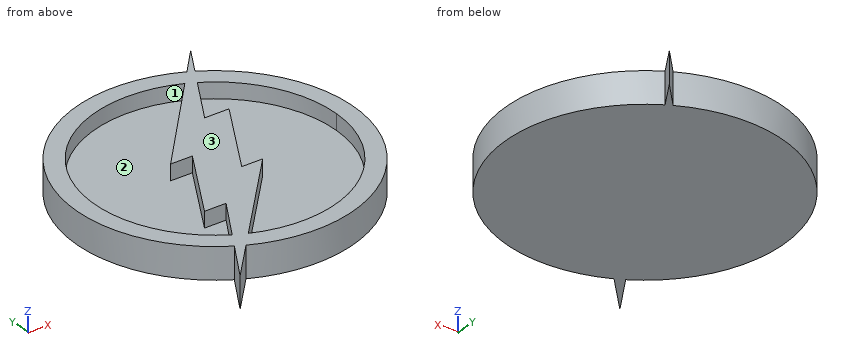
```python
from build123d import *

# Parameters (mm, degrees)
F1_DEPTH = 10.16
F2_DEPTH = 5.08


with BuildPart() as f1:
    # F0 (on Top) → F1 (new body)
    with BuildSketch(Plane.XY):
        with BuildLine():
            ThreePointArc((19.8948644209, 39.9997688602), (20.8320918018, 39.5197556971), (21.7577454104, 39.0177863782))
            Line((21.7577454104, 39.0177863782), (26.9711147994, 48.1350496411))
            Line((26.9711147994, 48.1350496411), (19.8948644209, 39.9997688602))
        make_face()
        with BuildLine():
            Line((-29.5520797372, -52.0064979792), (-19.2228405766, -40.327032365))
            ThreePointArc((-19.2228405766, -40.327032365), (-20.5915769431, -39.6456062912), (-21.9361932063, -38.9177410292))
            Line((-21.9361932063, -38.9177410292), (-29.5520797372, -52.0064979792))
        make_face()
        with BuildLine():
            ThreePointArc((-19.2228405766, -40.327032365), (23.8434631573, -37.7793118501), (44.6742335043, 0))
            ThreePointArc((44.6742335043, 0), (38.5214079324, 22.624947958), (21.7577454104, 39.0177863782))
            Line((21.7577454104, 39.0177863782), (18.8999443356, 34.0199965021))
            ThreePointArc((18.8999443356, 34.0199965021), (33.5418077285, 19.7361392424), (38.9174518423, 0))
            ThreePointArc((38.9174518423, 0), (21.4688277759, -32.460090755), (-15.2308770921, -35.8132439315))
            Line((-15.2308770922, -35.8132439315), (-19.2228405766, -40.327032365))
        make_face()
        with BuildLine():
            Line((18.8999443356, 34.0199965021), (21.7577454104, 39.0177863782))
            ThreePointArc((21.7577454104, 39.0177863782), (20.8320918018, 39.5197556971), (19.8948644209, 39.9997688602))
            Line((19.8948644209, 39.9997688602), (15.971442641, 35.4891684583))
            ThreePointArc((15.971442641, 35.4891684583), (17.4511611069, 34.7854140972), (18.8999443356, 34.0199965021))
        make_face()
        with BuildLine():
            ThreePointArc((-21.9361932063, -38.9177410292), (-20.5915769431, -39.6456062912), (-19.2228405766, -40.327032365))
            Line((-19.2228405766, -40.327032365), (-15.2308770922, -35.8132439315))
            ThreePointArc((-15.2308770921, -35.8132439315), (-17.1613070553, -34.9293228971), (-19.0406590573, -33.9414401662))
            Line((-19.0406590573, -33.9414401662), (-21.9361932063, -38.9177410292))
        make_face()
        with BuildLine():
            Line((9.9367275834, 18.344911789), (18.8999443356, 34.0199965021))
            ThreePointArc((18.8999443356, 34.0199965021), (17.4511611069, 34.7854140972), (15.971442641, 35.4891684583))
            Line((15.971442641, 35.4891684583), (-10.9691135585, 4.5166932978))
            Line((-10.9691135585, 4.5166932978), (-4.0004979819, 4.5166932978))
            Line((-4.0004979819, 4.5166932978), (-17.8778032411, -20.0695820685))
            Line((-17.8778032411, -20.0695820685), (-10.9691135585, -20.0695820685))
            Line((-10.9691135585, -20.0695820685), (-19.0406590573, -33.9414401662))
            ThreePointArc((-19.0406590573, -33.9414401662), (-17.1613070553, -34.9293228971), (-15.2308770921, -35.8132439315))
            Line((-15.2308770922, -35.8132439315), (9.9367275834, -7.3557584547))
            Line((9.9367275834, -7.3557584547), (3.2262078021, -7.3557584547))
            Line((3.2262078021, -7.3557584547), (17.7325143094, 18.344911789))
            Line((17.7325143094, 18.344911789), (9.9367275834, 18.344911789))
        make_face()
        with BuildLine():
            Line((15.971442641, 35.4891684583), (19.8948644209, 39.9997688602))
            ThreePointArc((19.8948644209, 39.9997688602), (-39.4719533034, 20.9225247427), (-21.9361932063, -38.9177410292))
            Line((-21.9361932063, -38.9177410292), (-19.0406590573, -33.9414401662))
            ThreePointArc((-19.0406590573, -33.9414401662), (-34.7492068376, 17.5231470361), (15.971442641, 35.4891684583))
        make_face()
    extrude(amount=F1_DEPTH)

    # F0 (on Top) → F2 (join)
    with BuildSketch(Plane.XY):
        with BuildLine():
            Line((-10.9691135585, 4.5166932978), (15.971442641, 35.4891684583))
            ThreePointArc((15.971442641, 35.4891684583), (-34.7492068376, 17.5231470361), (-19.0406590573, -33.9414401662))
            Line((-19.0406590573, -33.9414401662), (-10.9691135585, -20.0695820685))
            Line((-10.9691135585, -20.0695820685), (-17.8778032411, -20.0695820685))
            Line((-17.8778032411, -20.0695820685), (-4.0004979819, 4.5166932978))
            Line((-4.0004979819, 4.5166932978), (-10.9691135585, 4.5166932978))
        make_face()
        with BuildLine():
            ThreePointArc((38.9174518423, 0), (33.5418077285, 19.7361392424), (18.8999443356, 34.0199965021))
            Line((18.8999443356, 34.0199965021), (9.9367275834, 18.344911789))
            Line((9.9367275834, 18.344911789), (17.7325143094, 18.344911789))
            Line((17.7325143094, 18.344911789), (3.2262078021, -7.3557584547))
            Line((3.2262078021, -7.3557584547), (9.9367275834, -7.3557584547))
            Line((9.9367275834, -7.3557584547), (-15.2308770922, -35.8132439315))
            ThreePointArc((-15.2308770921, -35.8132439315), (21.4688277759, -32.460090755), (38.9174518423, 0))
        make_face()
    extrude(amount=F2_DEPTH)


solid = f1.part
```
Geometry check sheet. Reference: the model listing, model coordinates, mm. Face numbers are marked on the shaded views. Round coordinates to 2 decimals unless told otherwise and drop trailing zeros. Order: outer loops, then holes, each group sorted by start corner. A loop starts at its lowest first (then second) coordinate and runs counter-clockwise, first axis right, second up. Notation, with made-up numbers: (38.25, -31.5) - (81.25, -31.5) arc R24 cw to (81.25, -12.5) - close; hole circle Ø5 at (-16.75, 18). An arc over 180 degrees is marked (long way). Use a Markdown table: item, result. Add a question column.
(1) Release check for a two-part mould opening along X. For the marked faces 1, 2 and 3 record: pulls with the +X half, pulls with the -X half, needs draft (parallel to the pull), parting line crosses it, or undercut.
(2) Material ranges on line 1 along X through (y, z) = (-21.5, 7.25); line 2 along X through (y, z) = (6, 6.5); line 3 along Y through (x, z) = (14, 7.25), recorded low to high. Write a range as [from, to].
(3) Sectioned sample at D-D, the plane y = 29.5. Enter the section's corners in (x, z), and give its area (3 significant figures).
(4) Sectioned sample at B-B, the plane x = -24. Enter the section's corners in (y, z).
(5) Sectioned sample at C-C, the plane y = -43.5. Enter the section's corners in (x, z).
(6) Depth check by flat-ended pin: pin 1 (2.5 mm diameter, centred on x = 7, z = 7.5, fed in from +Y); pin 2 (1.5 mm diameter, centred on y = 12, z = 5.5, fed in from +X); pin 3 (1.5 mm diameter, centred on x = -8, z = 8, fed in from -Y); pin 4 (1 mm diameter, centred on x = 17.5, y = 21, fed in from -Z). Enter the tip coordinate at first touch or a pass-through.
Answers below:
| question | item | result |
|---|---|---|
| 1 | face 1 | undercut |
| 1 | face 2 | undercut |
| 1 | face 3 | needs draft |
| 2 | line 1 | [-39.16, -32.44], [-11.8, -2.57], [32.44, 39.16] |
| 2 | line 2 | [-44.27, -38.45], [-9.68, 10.76], [38.45, 44.27] |
| 2 | line 3 | [-42.42, -36.31], [11.73, 18.34], [25.45, 33.22], [36.31, 42.42] |
| 3 | outline | (-33.55, 0) - (33.55, 0) - (33.55, 10.16) - (25.38, 10.16) - (25.38, 5.08) - (16.32, 5.08) - (16.32, 10.16) - (10.76, 10.16) - (10.76, 5.08) - (-25.38, 5.08) - (-25.38, 10.16) - (-33.55, 10.16) - close |
| 3 | area | 452 mm² |
| 4 | outline | (-45.73, 0) - (-42.46, 0) - (-42.46, 10.16) - (-45.73, 10.16) - close; (-37.68, 0) - (37.68, 0) - (37.68, 10.16) - (30.64, 10.16) - (30.64, 5.08) - (-30.64, 5.08) - (-30.64, 10.16) - (-37.68, 10.16) - close |
| 5 | outline | (-24.6, 0) - (-22.03, 0) - (-22.03, 10.16) - (-24.6, 10.16) - close; (-10.18, 0) - (10.18, 0) - (10.18, 10.16) - (-10.18, 10.16) - close |
| 6 | pin 1 | y = 44.3 |
| 6 | pin 2 | x = 43.23 |
| 6 | pin 3 | y = -44.08 |
| 6 | pin 4 | z = 0 |
